```python
from build123d import *

# Parameters (mm, degrees)
BOSS_EXTRUDE1_DEPTH = 7.5
SKETCH3_R           = 16.5
BOSS_EXTRUDE2_DEPTH = 2.5
SKETCH6_R           = 5
CUT_EXTRUDE1_DEPTH  = 10
SKETCH7_R           = 5
BOSS_EXTRUDE3_DEPTH = 10


with BuildPart() as part:
    # Sketch1 → Boss-Extrude1 (new body, symmetric)
    with BuildSketch(Plane.XY):
        with BuildLine():
            Line((-81.983854392, -19.771263634), (88.350129521, -14.621102291))
            ThreePointArc((88.350129521, -14.621102291), (99.92815548, 1.466347152), (85.441176471, 14.993510707))
            Line((85.441176471, 14.993510707), (-84.411764706, 19.991347609))
            ThreePointArc((-84.411764706, 19.991347609), (-104.962820533, -1.218932468), (-81.983854392, -19.771263634))
        make_face()
    extrude(amount=BOSS_EXTRUDE1_DEPTH, both=True)

    # Sketch3 → Boss-Extrude2 (add, symmetric)
    with BuildSketch(Plane.XY.offset(7.5)):
        with Locations((-85, 0)):
            Circle(SKETCH3_R)
    extrude(amount=BOSS_EXTRUDE2_DEPTH, both=True)

    # Sketch6 → Cut-Extrude1 (cut)
    with BuildSketch(Plane.XY.offset(7.5)):
        with Locations((85, 0)):
            Circle(SKETCH6_R)
    extrude(amount=-CUT_EXTRUDE1_DEPTH, mode=Mode.SUBTRACT)

    # Sketch7 → Boss-Extrude3 (add)
    with BuildSketch(Plane(origin=(0, 0, -7.5), x_dir=(-1, 0, 0), z_dir=(0, 0, -1))):
        with Locations((85, 0)):
            Circle(SKETCH7_R)
    extrude(amount=BOSS_EXTRUDE3_DEPTH)


solid = part.part
```
Geometry check sheet. Reference: the model listing, model coordinates, mm. A direction names the side the tool comes from. Coordinates: 2 decimals unless noted, no trailing zeros. Loops run counter-clockwise (first coordinate to the right, second up) from the corner with the lowest first, then second, coordinate; pieces in that order, holes last. Notation, with made-up numbers: (-19.75, 88.5) -> (37.25, 88.5) arc R24 ccw to (37.25, 116.5) -> close; hole circle Ø7 at (77.5, 81). An arc over 180 degrees is marked (long way). Put each result on its own line as item: value.
1) Tool access check on faces 1 (the cylindrical face through (89.619, -1.915, 2.57)), 2 (the cylindrical face through (-89.619, -1.915, -12.43)), 3 (the flat face through (-85, 0, -17.5)). Record the directions out of +Z, -Z, +X, -X, +Y, -Y that give a thin tool (end or side, any length) a straight path to the whole face; none if there is none.
Result set:
face 1: +Z
face 2: -Z
face 3: -Z, +X, -X, +Y, -Y
2) Cross-section at B-B on z = -15.5. Record the boundary of the cut face in (x, y).
Result set:
outline: circle Ø10 at (-85, 0)
3) Gauge pin test, flat ends, axial feed: pin 1 Ø8 at (x, y) = (-69, -14) entering from -Z; pin 2 Ø12 at (y, z) = (10, -2.5) entering from +X; pin 3 Ø6 at (x, y) = (52, -0.5) entering from +Z. Record the tip position at first contact, or that the pin passes through.
Result set:
pin 1: stops at z = -7.5
pin 2: stops at x = 99.46
pin 3: stops at z = 7.5
4) Cross-section at A-A on y = 0. Record the boundary of the cut face in (x, z).
Result set:
outline: (-105, -7.5) -> (-90, -7.5) -> (-90, -17.5) -> (-80, -17.5) -> (-80, -7.5) -> (100, -7.5) -> (100, 7.5) -> (90, 7.5) -> (90, -2.5) -> (80, -2.5) -> (80, 7.5) -> (-68.5, 7.5) -> (-68.5, 10) -> (-101.5, 10) -> (-101.5, 7.5) -> (-105, 7.5) -> close
5) Release check for a two-part mould opening along X. For faces 4 (the cylindrical face through (-97.16, 11.15, 8.77)), 5 (the flat face through (-4, 0, 7.5)), 6 (the flat face through (85, 0, -2.5)), 7 (the cylindrical face through (99.955, 1.164, 0.105)) record: released by +X, released by -X, zero draft, split by the parting line, or undercut.
Result set:
face 4: split by the parting line
face 5: zero draft
face 6: undercut
face 7: released by +X
6) Cross-section at C-C on x = -47. Record the boundary of the cut face in (y, z), plus the area to 3 significant figures.
Result set:
outline: (-18.71, -7.5) -> (18.89, -7.5) -> (18.89, 7.5) -> (-18.71, 7.5) -> close
area: 564 mm^2
7) Cross-section at D-D on y = 11. Record the boundary of the cut face in (x, z), plus the area to 3 significant figures.
Result set:
outline: (-101.7, -7.5) -> (95.2, -7.5) -> (95.2, 7.5) -> (-72.7, 7.5) -> (-72.7, 10) -> (-97.3, 10) -> (-97.3, 7.5) -> (-101.7, 7.5) -> close
area: 3,020 mm^2
8) Thickness scan on line 1 (Y direction, x = -84, z = 3.75); line 2 (Z direction, x = -53.5, y = 2); line 3 (Y direction, x = 85, z = 0.5). Record the ranges inside material, lowest first.
Result set:
line 1: y = -19.97 to 19.98
line 2: z = -7.5 to 7.5
line 3: y = -14.72 to -5, 5 to 15.01
